```python
from build123d import *

# Parameters (mm, degrees)
SKETCH1_W           = 114.1727
SKETCH1_H           = 180
BOSS_EXTRUDE1_DEPTH = 3
SKETCH2_W           = 17.167528572
SKETCH2_H           = 3
SKETCH2_W_2         = 3
SKETCH2_H_2         = 20
BOSS_EXTRUDE2_DEPTH = 3
CUT_EXTRUDE1_DEPTH  = 10


with BuildPart() as part:
    # Sketch1 → Boss-Extrude1 (new body)
    with BuildSketch(Plane(origin=(0, 0, 0), x_dir=(0, 0, -1), z_dir=(1, 0, 0))):
        Rectangle(SKETCH1_W, SKETCH1_H)
    extrude(amount=BOSS_EXTRUDE1_DEPTH)

    # Sketch2 → Boss-Extrude2 (add)
    with BuildSketch(Plane(origin=(3, 0, 0), x_dir=(0, 0, -1), z_dir=(1, 0, 0))):
        with Locations((-34.335057143, -91.5)):
            Rectangle(SKETCH2_W, SKETCH2_H)
        with Locations((0, -91.5)):
            Rectangle(SKETCH2_W, SKETCH2_H)
        with Locations((34.335057143, -91.5)):
            Rectangle(SKETCH2_W, SKETCH2_H)
        with Locations((58.58635, -60)):
            Rectangle(SKETCH2_W_2, SKETCH2_H_2)
        with Locations((58.58635, -20)):
            Rectangle(SKETCH2_W_2, SKETCH2_H_2)
        with Locations((58.58635, 20)):
            Rectangle(SKETCH2_W_2, SKETCH2_H_2)
        with Locations((58.58635, 60)):
            Rectangle(SKETCH2_W_2, SKETCH2_H_2)
        with Locations((-58.58635, -60)):
            Rectangle(SKETCH2_W_2, SKETCH2_H_2)
        with Locations((-58.58635, -20)):
            Rectangle(SKETCH2_W_2, SKETCH2_H_2)
        with Locations((-58.58635, 20)):
            Rectangle(SKETCH2_W_2, SKETCH2_H_2)
        with Locations((-58.58635, 60)):
            Rectangle(SKETCH2_W_2, SKETCH2_H_2)
    extrude(amount=-BOSS_EXTRUDE2_DEPTH)

    # Sketch3 → Cut-Extrude1 (cut)
    with BuildSketch(Plane(origin=(0, 0, -3), x_dir=(0, 0, 1), z_dir=(-1, 0, 0))):
        Polygon((-25.867513459, -43), (-45.08635, -43), (-45.08635, -78), (-25.867513459, -78), (-15.763883749, -60.5), align=None)
        Polygon((-7.103629711, -65.5), (-14.320508076, -78), (20.320508076, -78), (13.103629711, -65.5), align=None)
        Polygon((21.763883749, -60.5), (31.867513459, -78), (51.08635, -78), (51.08635, -43), (31.867513459, -43), align=None)
        Polygon((23.207259422, -38), (13.103629711, -20.5), (-7.103629711, -20.5), (-17.207259422, -38), (-7.103629711, -55.5), (13.103629711, -55.5), align=None)
        Polygon((-45.08635, 2), (-45.08635, -33), (-25.867513459, -33), (-15.763883749, -15.5), (-25.867513459, 2), align=None)
        Polygon((23.207259422, 7), (13.103629711, 24.5), (-7.103629711, 24.5), (-17.207259422, 7), (-7.103629711, -10.5), (13.103629711, -10.5), align=None)
        Polygon((31.867513459, -33), (51.08635, -33), (51.08635, 2), (31.867513459, 2), (21.763883749, -15.5), align=None)
        Polygon((51.08635, 12), (51.08635, 47), (31.867513459, 47), (21.763883749, 29.5), (31.867513459, 12), align=None)
        Polygon((-45.08635, 47), (-45.08635, 12), (-25.867513459, 12), (-15.763883749, 29.5), (-25.867513459, 47), align=None)
        Polygon((23.207259422, 52), (13.103629711, 69.5), (-7.103629711, 69.5), (-17.207259422, 52), (-7.103629711, 34.5), (13.103629711, 34.5), align=None)
        Polygon((-45.08635, 78), (-45.08635, 57), (-25.867513459, 57), (-15.763883749, 74.5), (-17.784609691, 78), align=None)
        Polygon((51.08635, 78), (23.784609691, 78), (21.763883749, 74.5), (31.867513459, 57), (51.08635, 57), align=None)
    extrude(amount=-CUT_EXTRUDE1_DEPTH, mode=Mode.SUBTRACT)


solid = part.part
```
Here's how the part is built. I have some questions about the finished solid (model axes, mm). Coordinates: 2 decimals unless noted, no trailing zeros. Order: outer loops, then holes, each group sorted by start corner. A loop starts at its lowest first (then second) coordinate and runs counter-clockwise, first axis right, second up. Notation, with made-up numbers: (56.25, 4) -> (103.25, 4) arc R17 ccw to (103.25, 31) -> close; hole circle Ø1 at (7, 68). An arc over 180 degrees is marked (long way). Return JSON: item names as keys, results as strings.
1) Thinking about a two-plate mould opening in Y: for faces 1 (the flat face through (0, -21, -13)), 2 (the flat face through (1.479, -46.872, 15.085)), which applies, +Y half, -Y half, draft (parallel to the pull), parting line (faces both ways), or undercut?
Conclusion:
{"face 1": "draft", "face 2": "undercut"}
2) If we section it at D-D on z = -15: List the corners of the cut face in (x, y) for me.
Conclusion:
{"outline": "(0, -90) -> (3, -90) -> (3, -78) -> (0, -78) -> close; (0, -73.98) -> (3, -73.98) -> (3, -47.02) -> (0, -47.02) -> close; (0, -28.98) -> (3, -28.98) -> (3, -2.02) -> (0, -2.02) -> close; (0, 16.02) -> (3, 16.02) -> (3, 42.98) -> (0, 42.98) -> close; (0, 61.02) -> (3, 61.02) -> (3, 90) -> (0, 90) -> close"}
3) If I drill on probe 1 along Z at (x, y) = (1.3, -60.5); probe 2 along Y at (x, z) = (2.7, 34); probe 3 along Y at (x, z) = (0.2, -8), over which ranges is the centre line in solid material (lowest first)?
Conclusion:
{"probe 1": "z = -60.09 to -48.09, -18.76 to 18.76, 48.09 to 60.09", "probe 2": "y = -93 to -78, -43 to -33, 2 to 12, 47 to 57, 78 to 90", "probe 3": "y = -93 to -78, -65.5 to -55.5, -20.5 to -10.5, 24.5 to 34.5, 69.5 to 90"}
4) I'm going to push flat-ended pins straight in: P1, Ø1.5, axis at x = 2, z = 58, coming from the -Y side; P2, Ø1.5, axis at x = 1, y = 8.5, coming from the +Z side; P3, Ø0.9, axis at x = 1.5, z = 58.5, coming from the +Y side. Where does each tip first touch, or does it pass through?
Conclusion:
{"P1": "stops at y = -70", "P2": "stops at z = 57.09", "P3": "stops at y = 70"}
5) If we section it at B-B on z = 3.5: List the corners of the cut face in (x, y) for me.
Conclusion:
{"outline": "(0, -93) -> (3, -93) -> (3, -78) -> (0, -78) -> close; (0, -65.5) -> (3, -65.5) -> (3, -55.5) -> (0, -55.5) -> close; (0, -20.5) -> (3, -20.5) -> (3, -10.5) -> (0, -10.5) -> close; (0, 24.5) -> (3, 24.5) -> (3, 34.5) -> (0, 34.5) -> close; (0, 69.5) -> (3, 69.5) -> (3, 90) -> (0, 90) -> close"}
6) If we section it at C-C on y = 65.5: List the corners of the cut face in (x, z) for me, plus the area to 3 significant figures.
Conclusion:
{"outline": "(0, -60.09) -> (3, -60.09) -> (3, -48.09) -> (0, -48.09) -> close; (0, -23.96) -> (3, -23.96) -> (3, -12.41) -> (0, -12.41) -> close; (0, 12.41) -> (3, 12.41) -> (3, 23.96) -> (0, 23.96) -> close; (0, 48.09) -> (3, 48.09) -> (3, 60.09) -> (0, 60.09) -> close", "area": "141 mm²"}
7) If we section it at A-A on y = -35.5: List the corners of the cut face in (x, z) for me.
Conclusion:
{"outline": "(0, -57.09) -> (3, -57.09) -> (3, -18.76) -> (0, -18.76) -> close; (0, 18.76) -> (3, 18.76) -> (3, 57.09) -> (0, 57.09) -> close"}
